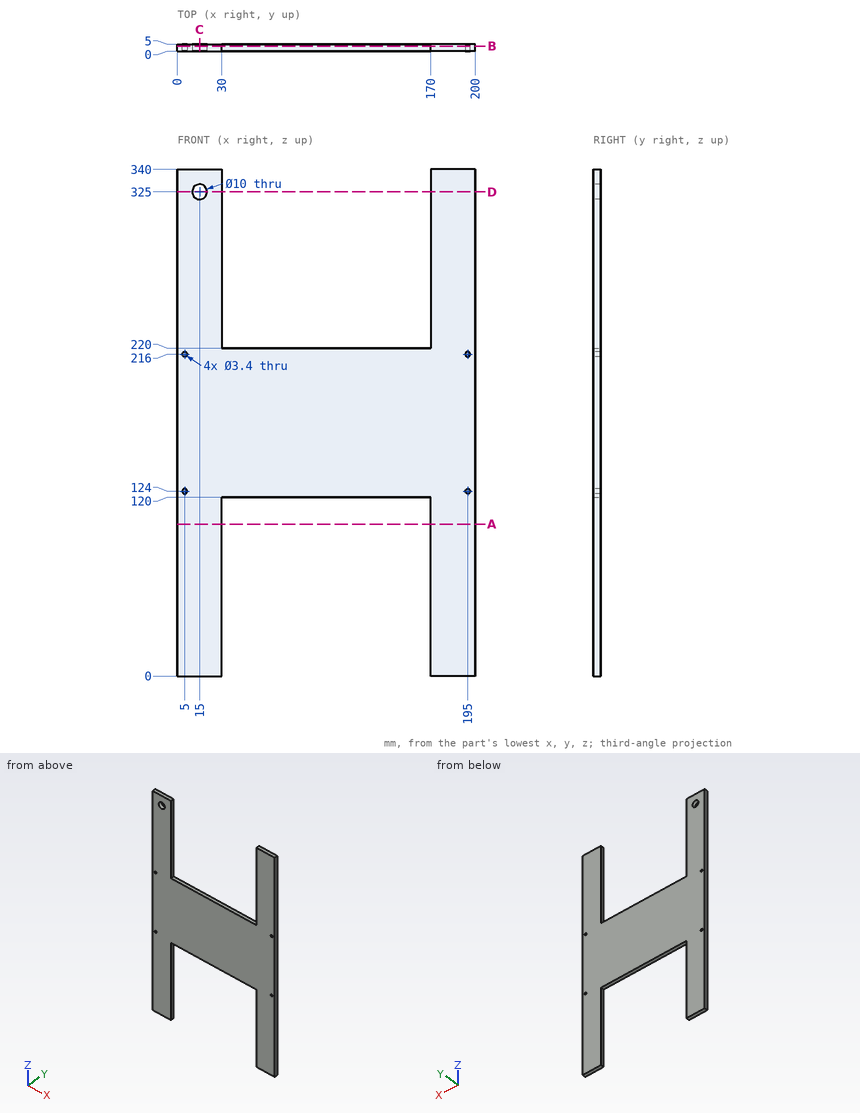
Verification items for this drawing (mm, ordinates from the low corner). Give positions to 0.01 mm unless a question says otherwise; leave off trailing zeros. Write each loop counter-clockwise with the first axis right and the second up, starting at its lowest first coordinate (ties: lowest second). Pieces come first, ordered by that corner, then holes. Notation, with made-up numbers: (7, -38) -> (47, -38) arc R22 cw to (47, -16) -> close; hole circle Ø9 at (-9, 25.25). An arc over 180 degrees is marked (long way). Use CSV: the item, a comma, the result in double quotes.
(1) Sectioned sample at D-D (z = 325). Record the cut outline in (x, y).
Derived:
outline,"(0, 0) -> (10, 0) -> (10, 5) -> (0, 5) -> close; (20, 0) -> (30, 0) -> (30, 5) -> (20, 5) -> close; (170, 0) -> (200, 0) -> (200, 5) -> (170, 5) -> close"
(2) Sectioned sample at C-C (x = 15). Record the cut outline in (y, z).
Derived:
outline,"(0, 0) -> (5, 0) -> (5, 320) -> (0, 320) -> close; (0, 330) -> (5, 330) -> (5, 340) -> (0, 340) -> close"
(3) Go/stop test with a flat-tipped pin: pin 1 (1.5 mm diameter, centred on x = 132.5, y = 2, fed in from -Z). Record where the tip stops, or that it passes through.
Derived:
pin 1,"stops at z = 120"
(4) Sectioned sample at B-B (y = 3.65). Record the cut outline in (x, z), plus the area to 3 significant figures.
Derived:
outline,"(0, 0) -> (30, 0) -> (30, 120) -> (170, 120) -> (170, 0) -> (200, 0) -> (200, 340) -> (170, 340) -> (170, 220) -> (30, 220) -> (30, 340) -> (0, 340) -> close; hole circle Ø3.4 at (5, 124); hole circle Ø3.4 at (5, 216); hole circle Ø10 at (15, 325); hole circle Ø3.4 at (195, 124); hole circle Ø3.4 at (195, 216)"
area,"34,300 mm^2"
(5) Material ranges on L1, parallel to Z at x = 5, y = 2.4; L2, parallel to X at y = 1.2, z = 216; L3, parallel to X at y = 3.15, z = 325, recorded low to high.
Derived:
L1,"z = 0 to 122.3, 125.7 to 214.3, 217.7 to 340"
L2,"x = 0 to 3.3, 6.7 to 193.3, 196.7 to 200"
L3,"x = 0 to 10, 20 to 30, 170 to 200"
(6) Sectioned sample at A-A (z = 102). Record the cut outline in (x, y), plus the area to 3 significant figures.
Derived:
outline,"(0, 0) -> (30, 0) -> (30, 5) -> (0, 5) -> close; (170, 0) -> (200, 0) -> (200, 5) -> (170, 5) -> close"
area,"300 mm^2"
